Verification items for the finished model (mm, model axes). Coordinates: 2 decimals unless noted, no trailing zeros. Order: outer loops, then holes, each group sorted by start corner. A loop starts at its lowest first (then second) coordinate and runs counter-clockwise, first axis right, second up. Notation, with made-up numbers: M 77,32.25 L 117,32.25 A19 cw 117,50.25 Z; hole C -16,56 d5. An arc over 180 degrees is marked long. Return JSON: item names as keys, results as strings.
```python
from build123d import *

# Parameters (mm, degrees)
SKETCH1_R           = 1.5
SKETCH1_R_2         = 2
SKETCH1_W           = 36
SKETCH1_H           = 20
BOSS_EXTRUDE1_DEPTH = 2


with BuildPart() as part:
    # Sketch1 → Boss-Extrude1 (new body)
    with BuildSketch(Plane.XY):
        Polygon((36, 0), (60, 0), (60, 60), (36, 60), (36, 55), (24, 55), (24, 60), (0, 60), (0, 0), (24, 0), align=None)
        with Locations((3, 57)):
            Circle(SKETCH1_R, mode=Mode.SUBTRACT)
        with Locations((3, 43)):
            Circle(SKETCH1_R, mode=Mode.SUBTRACT)
        with Locations((57, 57)):
            Circle(SKETCH1_R, mode=Mode.SUBTRACT)
        with Locations((57, 43)):
            Circle(SKETCH1_R, mode=Mode.SUBTRACT)
        with Locations((57, 17)):
            Circle(SKETCH1_R, mode=Mode.SUBTRACT)
        with Locations((57, 3)):
            Circle(SKETCH1_R, mode=Mode.SUBTRACT)
        with Locations((3, 17)):
            Circle(SKETCH1_R, mode=Mode.SUBTRACT)
        with Locations((3, 3)):
            Circle(SKETCH1_R, mode=Mode.SUBTRACT)
        with Locations((6, 30)):
            Circle(SKETCH1_R_2, mode=Mode.SUBTRACT)
        with Locations((54, 30)):
            Circle(SKETCH1_R_2, mode=Mode.SUBTRACT)
        with Locations((30, 30)):
            Rectangle(SKETCH1_W, SKETCH1_H, mode=Mode.SUBTRACT)
    extrude(amount=BOSS_EXTRUDE1_DEPTH)


solid = part.part
```
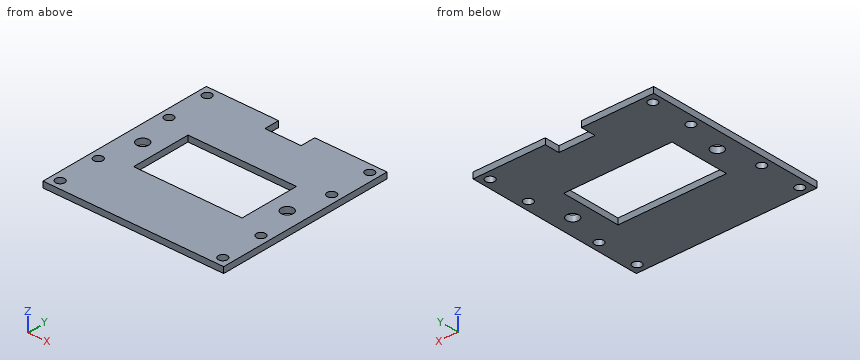
Q1. Material ranges on line 1 along Y through (x, z) = (57, 0.85); line 2 along Y through (x, z) = (32, 0.4); line 3 along X through (y, z) = (31.5, 0.6), recorded low to high.
Values:
{"line 1": "0 to 1.5, 4.5 to 15.5, 18.5 to 41.5, 44.5 to 55.5, 58.5 to 60", "line 2": "0 to 20, 40 to 55", "line 3": "0 to 4.68, 7.32 to 12, 48 to 52.68, 55.32 to 60"}
Q2. Cross-section at D-D, the plane x = 57. Record the boundary of the cut face in (y, z), and give its area (3 significant figures).
Values:
{"outline": "M 0,0 L 1.5,0 L 1.5,2 L 0,2 Z; M 4.5,0 L 15.5,0 L 15.5,2 L 4.5,2 Z; M 18.5,0 L 41.5,0 L 41.5,2 L 18.5,2 Z; M 44.5,0 L 55.5,0 L 55.5,2 L 44.5,2 Z; M 58.5,0 L 60,0 L 60,2 L 58.5,2 Z", "area": "96.0 mm^2"}
Q3. Cross-section at A-A, the plane y = 57. Record the boundary of the cut face in (x, z).
Values:
{"outline": "M 0,0 L 1.5,0 L 1.5,2 L 0,2 Z; M 4.5,0 L 24,0 L 24,2 L 4.5,2 Z; M 36,0 L 55.5,0 L 55.5,2 L 36,2 Z; M 58.5,0 L 60,0 L 60,2 L 58.5,2 Z"}
Q4. Go/stop test with flat-tipped pins: pin 1 (1.8 mm diameter, centred on x = 57, y = 3, fed in from -Z); pin 2 (0.6 mm diameter, centred on x = 28.5, z = 1, fed in from +Y). Record where each tip stops, or that it passes through.
Values:
{"pin 1": "through", "pin 2": "y = 55"}
Q5. Cross-section at B-B, the plane x = 38. Record the boundary of the cut face in (y, z).
Values:
{"outline": "M 0,0 L 20,0 L 20,2 L 0,2 Z; M 40,0 L 60,0 L 60,2 L 40,2 Z"}
Q6. Cross-section at C-C, the plane z = 1.15. State how many separate pieces and enclosed holes the cut face has, and give its area (3 significant figures).
Values:
{"separate pieces": "1", "enclosed holes": "11", "area": "2,740 mm^2"}
